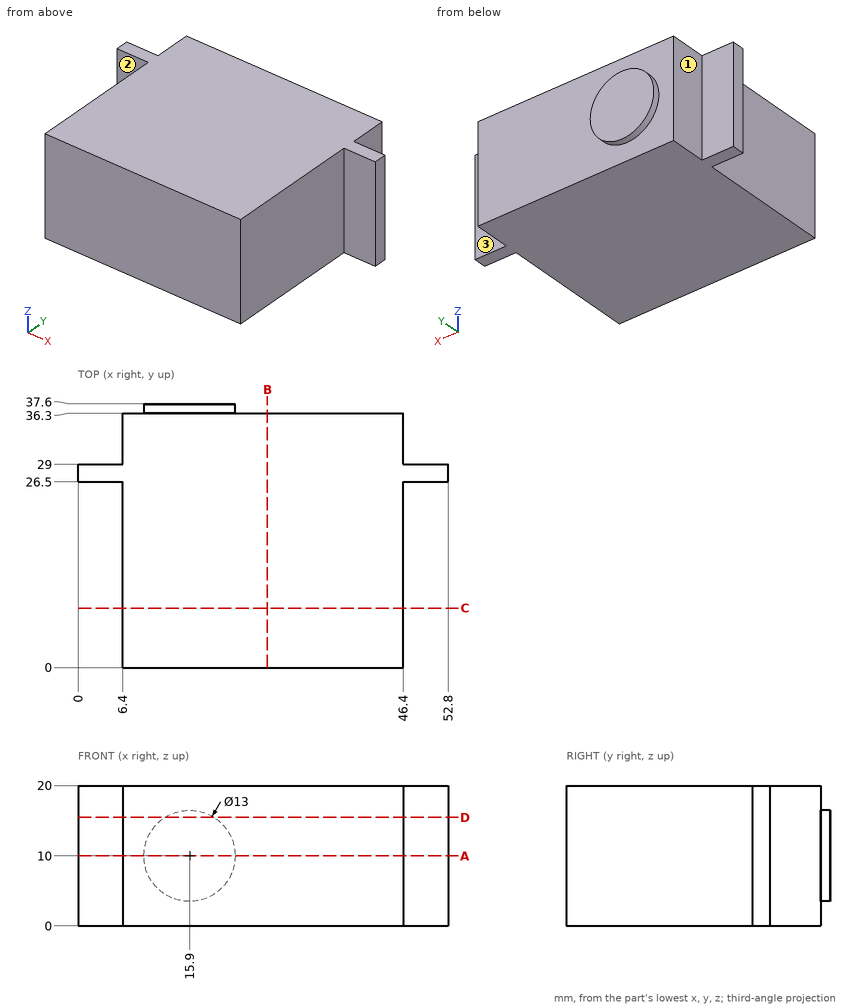
Geometry: see drawing. Coordinates: mm, zero at the bounding-box minimum. A direction names the side the tool comes from. Coordinates: 2 decimals unless noted, no trailing zeros. Order: outer loops, then holes, each group sorted by start corner. A loop starts at its lowest first (then second) coordinate and runs counter-clockwise, first axis right, second up. Notation, with made-up numbers: M 42.25,79.25 L 87.25,79.25 A35 ccw 87.25,115.25 Z; hole C 4,-7 d4. An arc over 180 degrees is marked long. Write item = value, one per line. Start each with the question number.
(1) Section D-D on z = 15.5. Output: boundary loops of the cut face in (x, y), and give its area (3 significant figures).
(2) Section B-B on x = 27. Output: boundary loops of the cut face in (y, z), and give its area (3 significant figures).
(3) Section A-A on z = 10. Output: boundary loops of the cut face in (x, y).
(4) Reachability of the marked faces 1, 2 and 3 from +Z, -Z, +X, -X, +Y, -Y: full face, straight path, thin tool, end or side. Return the list, or none.
(5) First-contact query: P1, Ø5, axis at x = 48, z = 7.5, coming from the +Y side; P2, Ø12, axis at x = 37.5, y = 6, coming from the -Z side; P3, Ø6, axis at y = 12.5, z = 2, coming from the -X side; P4, Ø5, axis at x = 51, z = 5, coming from the -Y side. Flat tips, straight axial feed; report the tip coordinate or a pass-through.
(6) Section C-C on y = 8.5. Output: boundary loops of the cut face in (x, z).
(7) Line query: line 1 along X through (y, z) = (17, 8.75); line 2 along Y through (x, z) = (9.5, 16.5). Output: solid intervals per line, ascending. Write a range as [from, to].
Result set:
q1.outline = M 0,26.5 L 6.4,26.5 L 6.4,0 L 46.4,0 L 46.4,26.5 L 52.8,26.5 L 52.8,29 L 46.4,29 L 46.4,36.3 L 19.36,36.3 L 19.36,37.6 L 12.44,37.6 L 12.44,36.3 L 6.4,36.3 L 6.4,29 L 0,29 Z
q1.area = 1,490 mm²
q2.outline = M 0,0 L 36.3,0 L 36.3,20 L 0,20 Z
q2.area = 726 mm²
q3.outline = M 0,26.5 L 6.4,26.5 L 6.4,0 L 46.4,0 L 46.4,26.5 L 52.8,26.5 L 52.8,29 L 46.4,29 L 46.4,36.3 L 22.4,36.3 L 22.4,37.6 L 9.4,37.6 L 9.4,36.3 L 6.4,36.3 L 6.4,29 L 0,29 Z
q4.face_1 = +Z, -Z, -X, +Y
q4.face_2 = +Z, -Z, -X, -Y
q4.face_3 = +Z, -Z, +X, +Y
q5.P1 = 36.3
q5.P2 = 0
q5.P3 = 6.4
q5.P4 = 26.5
q6.outline = M 6.4,0 L 46.4,0 L 46.4,20 L 6.4,20 Z
q7.line_1 = [6.4, 46.4]
q7.line_2 = [0, 36.3]
